The listing builds one solid part. Answer for the finished solid, in the listing's coordinates (mm). Give positions to 0.01 mm unless a question says otherwise; leave off trailing zeros. Write each loop counter-clockwise with the first axis right and the second up, starting at its lowest first coordinate (ties: lowest second). Pieces come first, ordered by that corner, then holes. Notation, with made-up numbers: M 6,57 L 44,57 A23 ccw 44,89 Z; hole C 20.5,-31 d10. An arc over 180 degrees is marked long. Answer as a JSON object with one key per item and string values.
```python
from build123d import *

# Parameters (mm, degrees)
F1_DEPTH = 12.7
F2_R     = 2.54
F4_DEPTH = 25.4


with BuildPart() as f1:
    # F0 (on Top) → F1 (new body)
    with BuildSketch(Plane.XY):
        with BuildLine():
            ThreePointArc((18.385943, -16.708252), (24.739692, -2.270726), (21.12025, 13.082187))
            Line((21.12025, 13.082187), (0, 36.817349))
            Line((0, 36.817349), (-37.818789, 76.065511))
            ThreePointArc((-37.818789, 76.065511), (-43.685006, 37.507391), (-32.992173, 0))
            ThreePointArc((-32.992173, 0), (-43.612045, -36.935455), (-37.818789, -74.928187))
            Line((-37.818789, -74.928187), (0, -36.940344))
            Line((0, -36.940344), (18.385943, -16.708252))
        make_face()
    extrude(amount=F1_DEPTH)

    # F2
    f2_edges = [f1.edges().sort_by_distance(p)[0] for p in [
        (-37.818789, -74.928187, 6.35),
        (-37.818789, 76.065511, 6.35),
    ]]
    fillet(f2_edges, radius=F2_R)

    # F3 (on face) → F4 (cut)
    with BuildSketch(Plane.XY.offset(12.7)):
        with BuildLine():
            ThreePointArc((18.385943, -16.708252), (24.739692, -2.270726), (21.12025, 13.082187))
            ThreePointArc((21.12025, 13.082187), (4.327566, -0.397205), (18.385943, -16.708252))
        make_face()
    extrude(amount=-F4_DEPTH, mode=Mode.SUBTRACT)


solid = f1.part
```
1. A cutting plane is placed at D-D, the plane x = -17. Give the vertices of the cut face in (y, z).
Verdict:
{"outline": "M -54.02,0 L 54.46,0 L 54.46,12.7 L -54.02,12.7 Z"}
2. The mould has two halves that part along Y. Classify faces 1 (the flat face through (-19, 2, 0)), 2 (the cylindrical face through (-43.573, 35.954, 6.261)), 3 (the flat face through (-17.24, 54.71, 6.26)): released by +Y, released by -Y, zero draft, split by the parting line, or undercut.
Verdict:
{"face 1": "zero draft", "face 2": "undercut", "face 3": "released by +Y"}
3. A cutting plane is placed at A-A, the plane x = 15. Give the vertices of the cut face in (y, z), plus the area to 3 significant figures.
Verdict:
{"outline": "M -20.43,0 L -16.12,0 L -16.12,12.7 L -20.43,12.7 Z; M 12.59,0 L 19.96,0 L 19.96,12.7 L 12.59,12.7 Z", "area": "148 mm2"}
4. A cutting plane is placed at C-C, the plane y = -51. Give the vertices of the cut face in (x, z), plus the area to 3 significant figures.
Verdict:
{"outline": "M -43.41,0 L -14,0 L -14,12.7 L -43.41,12.7 Z", "area": "374 mm2"}
5. Flat-ended cylindrical pins translate along their axes: pin 1 (4 mm diameter, centred on x = -12, y = -54.5, fed in from -Z); pin 2 (5 mm diameter, centred on x = -33, z = 9.5, fed in from -Y); pin 3 (1 mm diameter, centred on x = -30, z = 7.5, fed in from +Y); pin 4 (1.5 mm diameter, centred on y = 0, z = 3.5, fed in from +X). Find the tip coordinate at first contact, or state that the pin passes through.
Verdict:
{"pin 1": "passes through", "pin 2": "stops at y = -72.48", "pin 3": "stops at y = 68.47", "pin 4": "stops at x = 4.48"}
6. Consider line 1 along Y through (x, z) = (-33.5, 10.5); line 2 along X through (y, z) = (-32.5, 11.5); line 3 along X through (y, z) = (32.5, 10). Determine where each line is inside the solid, lowest interval first.
Verdict:
{"line 1": "y = -70.59 to -0.95, 0.96 to 71.58", "line 2": "x = -43.22 to 4.04", "line 3": "x = -43.23 to 3.84"}
7. A cutting plane is placed at B-B, the plane z = 6.5. Give the vertices of the cut face in (x, y).
Verdict:
{"outline": "M -39.22,72.15 A91.68 ccw -32.99,0 A89.8 ccw -39.19,-71.09 A2.54 ccw -34.98,-72.08 L 0,-36.94 L 18.39,-16.71 A14.97 cw long 21.12,13.08 L 0,36.82 L -34.98,73.11 A2.54 ccw Z"}
